Geometry: final body of the model. Coordinates: model frame, mm. Give positions to 0.01 mm unless a question says otherwise; leave off trailing zeros. Write each loop counter-clockwise with the first axis right and the second up, starting at its lowest first coordinate (ties: lowest second). Pieces come first, ordered by that corner, then holes.
```python
from build123d import *

# Parameters (mm, degrees)
F1_DEPTH = 10


with BuildPart() as f1:
    # F0 (on Front) → F1 (new body)
    with BuildSketch(Plane.XZ):
        with BuildLine():
            ThreePointArc((-19.814088, 0), (-24.397086, -4.014774), (-27.773799, 1.056724))
            Line((-27.773799, 1.056724), (-32.496632, -6))
            Line((-32.496632, -6), (-17.814088, -6))
            Line((-17.814088, -6), (-17.814088, 0))
            Line((-17.814088, 0), (-19.814088, 0))
        make_face()
        with BuildLine():
            Line((-15.814088, 0), (-17.814088, 0))
            Line((-17.814088, 0), (-17.814088, -6))
            Line((-17.814088, -6), (-3.131545, -6))
            Line((-3.131545, -6), (-7.854378, 1.056724))
            ThreePointArc((-7.854378, 1.056724), (-11.231091, -4.014774), (-15.814088, 0))
        make_face()
    extrude(amount=F1_DEPTH)


solid = f1.part
```
Item 1: Section A-A, the plane z = -3. Return the cut outline in (x, y).
Found:
outline: (-30.49, -10) - (-26.58, -10) - (-26.58, 0) - (-30.49, 0) - close; (-21.14, -10) - (-14.48, -10) - (-14.48, 0) - (-21.14, 0) - close; (-9.04, -10) - (-5.14, -10) - (-5.14, 0) - (-9.04, 0) - close
Item 2: Section D-D, the plane x = -24. Return the cut outline in (y, z).
Found:
outline: (-10, -6) - (0, -6) - (0, -4.05) - (-10, -4.05) - close
Item 3: Section B-B, the plane y = -9. Return the cut outline in (x, z).
Found:
outline: (-32.5, -6) - (-3.13, -6) - (-7.85, 1.06) arc R4.05 cw (long way) to (-15.81, 0) - (-19.81, 0) arc R4.05 cw (long way) to (-27.77, 1.06) - close
Item 4: Line query: L1, parallel to X at y = -3.5, z = -3.25; L2, parallel to X at y = -0.75, z = -3; L3, parallel to Z at x = -17.5, y = -7.25. Output: solid intervals per line, ascending.
Found:
L1: x = -30.66 to -26.28, -21.45 to -14.18, -9.35 to -4.97
L2: x = -30.49 to -26.58, -21.14 to -14.48, -9.04 to -5.14
L3: z = -6 to 0
Item 5: Pin query (flat end, axial travel): pin 1 Ø1.5 at (y, z) = (-1, -3.5) entering from +X; pin 2 Ø3 at (y, z) = (-3, -1.5) entering from +X; pin 3 Ø2 at (y, z) = (-5, -0.5) entering from -X. Return the tip coordinate at first contact, or that it passes through.
Found:
pin 1: stops at x = -4.3
pin 2: stops at x = -5.14
pin 3: stops at x = -29.48
Item 6: Pull-direction query (X, two-part tool) for faces 1 (the face through (-5.46, -4.93, -2.52)), 2 (the face through (-18, -5, 0)), 3 (the face through (-18, -5, -6)), 4 (the face through (-24.301, -4.93, -4.026)); classes: +X half, -X half, draft (parallel to the pull), parting line (faces both ways), or undercut.
Found:
face 1: +X half
face 2: undercut
face 3: draft
face 4: undercut
Item 7: Section C-C, the plane x = -12.25. Return the cut outline in (y, z).
Found:
outline: (-10, -6) - (0, -6) - (0, -4.02) - (-10, -4.02) - close
